The listing builds one solid part. Answer for the finished solid, in the listing's coordinates (mm). A direction names the side the tool comes from. Coordinates: 2 decimals unless noted, no trailing zeros. Order: outer loops, then holes, each group sorted by start corner. A loop starts at its lowest first (then second) coordinate and runs counter-clockwise, first axis right, second up. Notation, with made-up numbers: (30, 7.25) -> (80, 7.25) arc R22 cw to (80, 41.25) -> close; hole circle Ø5 at (9, -19.75). An arc over 180 degrees is marked (long way). Write item = value, one per line.
Autodesk Inventor part; units mm, degrees
ref_plane "YZ Plane" through (0, 0, 0) normal (1, 0, 0) x (0, 1, 0)
ref_plane "XZ Plane" through (0, 0, 0) normal (0, 1, 0) x (-1, 0, 0)
ref_plane "XY Plane" through (0, 0, 0) normal (0, 0, 1) x (1, 0, 0)
sketch "Sketch1" plane through (0, 0, 0) normal (0, 0, 1) x (1, 0, 0)
  line L0 (46.5, 31) -> (61.5, 31)
  line L1 (61.5, 31) -> (61.5, 11)
  line L2 (61.5, 11) -> (46.5, 11)
  line L3 (46.5, 11) -> (46.5, 31)
  circle A0 centre (60.5, 2.5) radius 1.5
  circle A1 centre (2.5, 2.5) radius 1.5
  line L4 (0, 9.4) -> (0, 0)
  line L5 (0, 0) -> (5, 0)
  line L6 (5, 0) -> (5, 3)
  line L7 (5, 3) -> (29, 3)
  line L8 (29, 3) -> (29, 0)
  line L9 (29, 0) -> (34, 0)
  line L10 (34, 0) -> (34, 3)
  line L11 (34, 3) -> (58, 3)
  line L12 (58, 3) -> (58, 0)
  line L13 (58, 0) -> (63, 0)
  line L14 (63, 0) -> (63, 32.5)
  line L15 (63, 32.5) -> (45, 32.5)
  line L16 (45, 32.5) -> (45, 9.4)
  line L17 (45, 9.4) -> (31, 9.4)
  line L18 (31, 9.4) -> (31, 7)
  line L19 (31, 7) -> (6, 7)
  line L20 (6, 7) -> (6, 9.4)
  line L21 (6, 9.4) -> (0, 9.4)
extrude "Extrusion1" add sketch "Sketch1" along normal blind 6
properties part number "yCarMid_d"
Q1. Section B-B, the plane x = 60.5 is taken. Give the vertices of the cut face in (y, z), plus the area to 3 significant figures.
The answers:
outline = (0, 0) -> (1, 0) -> (1, 6) -> (0, 6) -> close; (4, 0) -> (11, 0) -> (11, 6) -> (4, 6) -> close; (31, 0) -> (32.5, 0) -> (32.5, 6) -> (31, 6) -> close
area = 57.0 mm2
Q2. Each of these flat-tipped pins is pushed along its axis until it touches: pin 1 Ø3 at (x, z) = (4.5, 3.5) entering from +Y; pin 2 Ø2 at (x, z) = (21.5, 4.5) entering from +Y; pin 3 Ø1.8 at (y, z) = (26, 2.5) entering from -X. Where does it stop, or does it pass through?
The answers:
pin_1 = 9.4
pin_2 = 7
pin_3 = 45
Q3. A tool of negligible diameter and unlimited length cuts with its end or side. For faces 1 (the face through (31, 8, 3)), 2 (the face through (3, 9.4, 3)), 3 (the face through (46, 3, 3)), from which of +Z, -Z, +X, -X, +Y, -Y can it reach the whole face along a straight path? Write none if from no direction.
The answers:
face_1 = +Z, -Z, +Y
face_2 = +Z, -Z, -X, +Y
face_3 = +Z, -Z, -Y
Q4. Section C-C, the plane y = 29 is taken. Give the vertices of the cut face in (x, z).
The answers:
outline = (45, 0) -> (46.5, 0) -> (46.5, 6) -> (45, 6) -> close; (61.5, 0) -> (63, 0) -> (63, 6) -> (61.5, 6) -> close
Q5. Section D-D, the plane x = 2.5 is taken. Give the vertices of the cut face in (y, z), plus the area to 3 significant figures.
The answers:
outline = (0, 0) -> (1, 0) -> (1, 6) -> (0, 6) -> close; (4, 0) -> (9.4, 0) -> (9.4, 6) -> (4, 6) -> close
area = 38.4 mm2
Q6. The mould has two halves that part along X. Classify faces 4 (the face through (5, 1, 3)), 5 (the face through (60, 0, 3)), 6 (the face through (61.5, 21, 3)), 7 (the face through (0, 5, 3)): released by +X, released by -X, zero draft, split by the parting line, or undercut.
The answers:
face_4 = undercut
face_5 = zero draft
face_6 = undercut
face_7 = released by -X
Q7. Find the intervals of material crossed by line 1 along Y through (x, z) = (2.5, 4.1); line 2 along Y through (x, z) = (56, 5.35); line 3 along X through (y, z) = (21.5, 1.1), in increasing order.
The answers:
line_1 = 0 to 1, 4 to 9.4
line_2 = 3 to 11, 31 to 32.5
line_3 = 45 to 46.5, 61.5 to 63
Q8. Section A-A, the plane z = 3.7 is taken. Give the vertices of the cut face in (x, y).
The answers:
outline = (0, 0) -> (5, 0) -> (5, 3) -> (29, 3) -> (29, 0) -> (34, 0) -> (34, 3) -> (58, 3) -> (58, 0) -> (63, 0) -> (63, 32.5) -> (45, 32.5) -> (45, 9.4) -> (31, 9.4) -> (31, 7) -> (6, 7) -> (6, 9.4) -> (0, 9.4) -> close; hole circle Ø3 at (2.5, 2.5); hole (46.5, 11) -> (61.5, 11) -> (61.5, 31) -> (46.5, 31) -> close; hole circle Ø3 at (60.5, 2.5)
